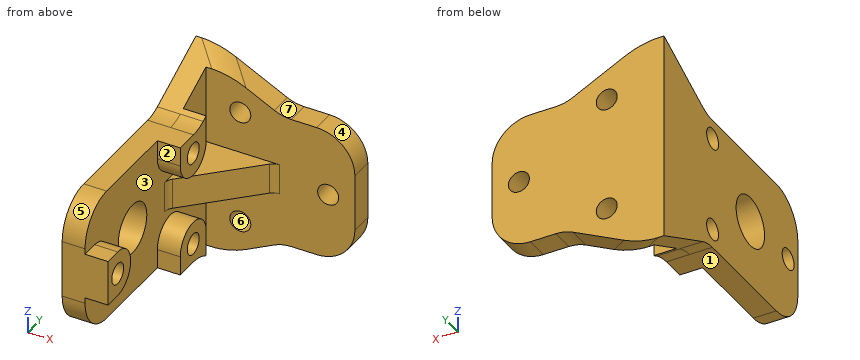
```python
from build123d import *

# Parameters (mm, degrees)
BOSS_EXTRUDE1_DEPTH  = 17.5
SKETCH2_R            = 6.6
CUT_EXTRUDE1_DEPTH   = 20
BOSS_EXTRUDE2_DEPTH  = 4
BOSS_EXTRUDE3_DEPTH  = 6
BOSS_EXTRUDE4_DEPTH  = 6
CUT_EXTRUDE2_DEPTH   = 8
FILLET3_R            = 10
FILLET4_R            = 3
M5_CLEARANCE_HOLE1_D = 5.5
FILLET5_R            = 10
BOSS_EXTRUDE5_START  = 6
BOSS_EXTRUDE5_DEPTH  = 6
M5_CLEARANCE_HOLE2_D = 5.5


with BuildPart() as part:
    # Sketch1 → Boss-Extrude1 (new, symmetric)
    with BuildSketch(Plane.XY):
        Polygon((0, -62), (0, 0), (45, 0), (45, -6), (6, -6), (6, -62), align=None)
    extrude(amount=BOSS_EXTRUDE1_DEPTH, both=True)

    # Sketch2 → Cut-Extrude1 (cut)
    with BuildSketch(Plane.ZY):
        with Locations((0, -40)):
            Circle(SKETCH2_R)
    extrude(amount=-CUT_EXTRUDE1_DEPTH, mode=Mode.SUBTRACT)

    # Sketch3 → Boss-Extrude2 (add, symmetric)
    with BuildSketch(Plane.XY):
        Polygon((6, -24), (24, -6), (6, -6), align=None)
    extrude(amount=BOSS_EXTRUDE2_DEPTH, both=True)

    # Sketch4 → Boss-Extrude3 (add)
    with BuildSketch(Plane.ZY):
        Polygon((17.5, -20), (27.5, 0), (17.5, 0), align=None)
    boss_extrude3 = extrude(amount=-BOSS_EXTRUDE3_DEPTH)

    # Sketch5 → Boss-Extrude4 (add)
    with BuildSketch(Plane(origin=(0, 0, 0), x_dir=(1, 0, 0), z_dir=(0, 1, 0))):
        Polygon((6, -27.5), (26, -17.5), (6, -17.5), align=None)
    boss_extrude4 = extrude(amount=-BOSS_EXTRUDE4_DEPTH)

    # Sketch6 → Cut-Extrude2 (cut)
    with BuildSketch(Plane.ZY.offset(-6)):
        Polygon((27.5, 0), (27.5, -6), (24.5, -6), align=None)
    cut_extrude2 = extrude(amount=-CUT_EXTRUDE2_DEPTH, mode=Mode.SUBTRACT)

    # Mirror2: Boss-Extrude3, Boss-Extrude4, Cut-Extrude2 across plane
    add(boss_extrude3.mirror(Plane.XY))
    add(boss_extrude4.mirror(Plane.XY))
    add(cut_extrude2.mirror(Plane.XY), mode=Mode.SUBTRACT)

    # Fillet3
    fillet3_edges = [part.edges().sort_by_distance(p)[0] for p in [
        (3, -20, 17.5),
        (26, -3, 17.5),
        (9, -3, 26),
        (3, -20, -17.5),
        (26, -3, -17.5),
        (9, -3, -26),
    ]]
    fillet(fillet3_edges, radius=FILLET3_R)

    # Fillet4
    fillet4_edges = [part.edges().sort_by_distance(p)[0] for p in [
        (6, -24, 0),
        (24, -6, 0),
    ]]
    fillet(fillet4_edges, radius=FILLET4_R)

    # M5 Clearance Hole1 (through all)
    with Locations(Plane(origin=(0, -6, 0), x_dir=(-1, 0, 0), z_dir=(0, -1, 0))):
        with Locations((-15, 15), (-15, -15), (-38, 0)):
            Hole(M5_CLEARANCE_HOLE1_D / 2)

    # Fillet5
    fillet5_edges = [part.edges().sort_by_distance(p)[0] for p in [
        (45, -3, 17.5),
        (3, -62, 17.5),
        (45, -3, -17.5),
        (3, -62, -17.5),
    ]]
    fillet(fillet5_edges, radius=FILLET5_R)

    # Sketch11 → Boss-Extrude5 (add)
    with BuildSketch(Plane(origin=(6, 0, 0), x_dir=(0, 0, -1), z_dir=(1, 0, 0)).offset(BOSS_EXTRUDE5_START)):
        with BuildLine():
            Line((17.5, -28.5), (17.5, -22.360679775))
            ThreePointArc((17.5, -22.360679775), (17.767510105, -20.06315057), (18.55572809, -17.88854382))
            Line((18.55572809, -17.88854382), (19.25, -16.5))
            Line((19.25, -16.5), (12.5, -16.5))
            ThreePointArc((12.5, -16.5), (6.5, -22.5), (12.5, -28.5))
            Line((12.5, -28.5), (17.5, -28.5))
        make_face()
        with BuildLine():
            Line((-17.5, -28.5), (-17.5, -22.360679775))
            ThreePointArc((-17.5, -22.360679775), (-17.767510105, -20.06315057), (-18.55572809, -17.88854382))
            Line((-18.55572809, -17.88854382), (-19.25, -16.5))
            Line((-19.25, -16.5), (-12.5, -16.5))
            ThreePointArc((-12.5, -16.5), (-6.5, -22.5), (-12.5, -28.5))
            Line((-12.5, -28.5), (-17.5, -28.5))
        make_face()
        with BuildLine():
            Line((-6, -57.5), (-6, -62))
            Line((-6, -62), (6, -62))
            Line((6, -62), (6, -57.5))
            ThreePointArc((6, -57.5), (0, -51.5), (-6, -57.5))
        make_face()
    extrude(amount=-BOSS_EXTRUDE5_DEPTH)

    # M5 Clearance Hole2 (through all)
    with Locations(Plane(origin=(12, 0, 0), x_dir=(0, 0, -1), z_dir=(1, 0, 0))):
        with Locations((-12.5, -22.5), (12.5, -22.5), (0, -57.5)):
            Hole(M5_CLEARANCE_HOLE2_D / 2)


solid = part.part
```
For this review, take the finished solid that the model builds, in its own axes (mm). Face numbers are marked on the shaded views. A direction names the side the tool comes from. Round coordinates to 2 decimals unless told otherwise and drop trailing zeros. Write each loop counter-clockwise with the first axis right and the second up, starting at its lowest first coordinate (ties: lowest second). Pieces come first, ordered by that corner, then holes. Notation, with made-up numbers: (19, 70) - (39, 70) arc R13 ccw to (39, 86) - close; hole circle Ø3 at (71.5, 20). An arc over 180 degrees is marked (long way). Answer as CSV lines item,"result". Start each with the question number.
(1) For line 1 (Y direction, x = 9, z = 12); line 2 (Y direction, x = 8.5, z = -17); line 3 (Y direction, x = 3, z = 0), list the stretches that pass through material, from the lowest coordinate up.
(2) Add section B-B, the plane x = 38. State the section outline as (y, z) points, plus the area to 3 significant figures.
(3) Add section D-D, the plane y = -21. State the section outline as (x, z) points.
(4) Add section C-C, the plane z = 13.5. State the section outline as (x, y) points, plus the area to 3 significant figures.
(5) For pin 1 (3 mm diameter, centred on x = 31.5, y = -4, fed in from +Z); pin 2 (1.3 mm diameter, centred on x = 7.5, y = -58.5, fed in from +Z); pin 3 (8.5 mm diameter, centred on y = -54, z = -1.5, fed in from +X), all flat-tipped, find the tip position at first contact; note any pin that passes through.
(6) Add section A-A, the plane z = 0. State the section outline as (x, y) points, plus the area to 3 significant figures.
(7) Mouldability with a two-part tool opening along X and no side actions: class the marked faces 5, 6 and 7 as +X half, -X half, draft (parallel to the pull), parting line (faces both ways), or undercut.
(8) Machinability: for the marked faces 1, 2, 3 and 4, which of the approach directions +Z, -Z, +X, -X, +Y, -Y give a long, thin tool a straight path to every point of the face, cutting with its end or side? Answer none if there is none.
From the geometry:
1,line 1,"y = -28.48 to -25.2, -19.8 to -16.52, -6 to 0"
1,line 2,"y = -28.5 to -16.5, -6 to 0"
1,line 3,"y = -62 to -60.25, -54.75 to -46.6, -33.4 to 0"
2,outline,"(-6, -17.04) - (0, -17.04) - (0, -2.75) - (-6, -2.75) - close; (-6, 2.75) - (0, 2.75) - (0, 17.04) - (-6, 17.04) - close"
2,area,"171 mm²"
3,outline,"(0, -17.59) - (12, -17.59) - (12, -14.8) - (0, -14.8) - close; (0, -10.2) - (12, -10.2) - (12, -6.69) - (6, -6.69) - (6, -4) - (9, -4) - (9, 4) - (6, 4) - (6, 6.69) - (12, 6.69) - (12, 10.2) - (0, 10.2) - close; (0, 14.8) - (12, 14.8) - (12, 17.59) - (0, 17.59) - close"
4,outline,"(0, -60) - (6, -60) - (6, -28.5) - (12, -28.5) - (12, -25.06) - (0, -25.06) - close; (0, -19.94) - (12, -19.94) - (12, -16.5) - (6, -16.5) - (6, -6) - (12.7, -6) - (12.7, 0) - (0, 0) - close; (17.3, -6) - (43, -6) - (43, 0) - (17.3, 0) - close"
4,area,"565 mm²"
5,pin 1,"stops at z = 17.5"
5,pin 2,"stops at z = 6"
5,pin 3,"stops at x = 12"
6,outline,"(0, -62) - (12, -62) - (12, -60.25) - (0, -60.25) - close; (0, -54.75) - (12, -54.75) - (12, -51.5) - (6, -51.5) - (6, -46.6) - (0, -46.6) - close; (0, -33.4) - (6, -33.4) - (6, -25.24) arc R3 cw to (6.88, -23.12) - (23.12, -6.88) arc R3 cw to (25.24, -6) - (35.25, -6) - (35.25, 0) - (0, 0) - close; (40.75, -6) - (45, -6) - (45, 0) - (40.75, 0) - close"
6,area,"653 mm²"
7,face 5,"draft"
7,face 6,"undercut"
7,face 7,"+X half"
8,face 1,"-Z, +X, -X, -Y"
8,face 2,"+Z, -Z, +X, -Y"
8,face 3,"+X"
8,face 4,"+Z, +X, +Y, -Y"
